Geometry: final body of the model. Coordinates: model frame, mm. Give positions to 0.01 mm unless a question says otherwise; leave off trailing zeros. Loops run counter-clockwise (first coordinate to the right, second up) from the corner with the lowest first, then second, coordinate; pieces in that order, holes last.
1. Material intervals for line 1 along X through (y, z) = (1, 0.45) (3 decimals); line 2 along Y through (x, z) = (1, 1.2) (3 decimals); line 3 along X through (y, z) = (35, 1.3) (3 decimals), sorted ascending.
2. Section A-A, the plane z = 1.6. Output: boundary loops of the cut face in (x, y) (3 decimals).
3. Section B-B, the plane x = 36.5. Output: boundary loops of the cut face in (y, z), then the cut area to 3 significant figures.
4. Draft query along Y for faces 1 (the face through (0, 25, 1)), 2 (the face through (20, 0, 1)), 3 (the face through (35.72, 45.49, 1.01)). Return one class per face: +Y half, -Y half, draft (parallel to the pull), parting line (faces both ways), or undercut.
5. Section C-C, the plane y = 41. Output: boundary loops of the cut face in (x, z), then the cut area to 3 significant figures.
Autodesk Inventor part; units mm, degrees
ref_plane "YZ Plane" through (0, 0, 0) normal (1, 0, 0) x (0, 1, 0)
ref_plane "XZ Plane" through (0, 0, 0) normal (0, 1, 0) x (-1, 0, 0)
ref_plane "XY Plane" through (0, 0, 0) normal (0, 0, 1) x (1, 0, 0)
sketch "Sketch1" plane through (0, 0, 0) normal (0, 0, 1) x (1, 0, 0)
  point P0 (0, 0)
sketch "Sketch2" plane through (0, 0, 0) normal (0, 0, 1) x (1, 0, 0)
  line L0 (0, 0) -> (40, 0)
  line L1 (40, 0) -> (40, 50)
  line L2 (40, 50) -> (0, 50)
  line L3 (0, 50) -> (0, 0)
extrude "Extrusion1" add sketch "Sketch2" along normal blind 2
sketch "Sketch3" plane through (0, 0, 2) normal (0, 0, 1) x (1, 0, 0)
  point P0 (0, 0)
fillet "Fillet1" radius 15 1 edges at (40, 50, 1)
sketch "Sketch4" plane through (0, 0, 2) normal (0, 0, 1) x (1, 0, 0)
  point P0 (0, 0)
  point P1 (1, 1)
  point P2 (39, 35)
hole "Hole1" at (1, 1, 2) direction (0, 0, -1) diameter 0.37 end through all
sketch "Sketch5" plane through (0, 0, 2) normal (0, 0, 1) x (1, 0, 0)
  point P0 (0, 0)
  point P1 (39, 35)
hole "Hole2" at (39, 35, 2) direction (0, 0, -1) diameter 0.37 end through all
properties part number "Dół"
Answers below:
1. line 1: x = 0 to 0.815, 1.185 to 40
1. line 2: y = 0 to 0.815, 1.185 to 50
1. line 3: x = 0 to 38.815, 39.185 to 40
2. outline: (0, 0) - (40, 0) - (40, 35) arc R15 ccw to (25, 50) - (0, 50) - close; hole circle Ø0.37 at (1, 1); hole circle Ø0.37 at (39, 35)
3. outline: (0, 0) - (44.63, 0) - (44.63, 2) - (0, 2) - close
3. area: 89.3 mm2
4. face 1: draft
4. face 2: -Y half
4. face 3: +Y half
5. outline: (0, 0) - (38.75, 0) - (38.75, 2) - (0, 2) - close
5. area: 77.5 mm2
